Geometry check sheet. Reference: the model listing, model coordinates, mm. Round coordinates to 2 decimals unless told otherwise and drop trailing zeros. Order: outer loops, then holes, each group sorted by start corner. A loop starts at its lowest first (then second) coordinate and runs counter-clockwise, first axis right, second up. Notation, with made-up numbers: (33, 32) -> (61, 32) arc R20 ccw to (61, 66) -> close; hole circle Ø5 at (13.5, 12). An arc over 180 degrees is marked (long way). Use a Markdown table: item, result. Add a question column.
Item 1: Material ranges on probe 1 along X at (y, z) = (0.6, 0); probe 2 along Z at (x, y) = (-4.75, 0.5), recorded low to high. Write a range as [from, to].
Item 2: Mould release check, pull along Z, two halves, no side actions. Record for faces 1 (the cylindrical face through (-6.834, 0.887, -1.517)), 2 (the cylindrical face through (3.604, 0.99, 11.446)), 3 (the flat face through (-5.1, 0, 5.1)): pulls with the +Z half, pulls with the -Z half, needs draft (parallel to the pull), parting line crosses it, or undercut.
Item 3: Sectioned sample at B-B, the plane z = 0. Record the cut outline in (x, y).
Item 4: Gauge pin test, flat ends, axial feed: pin 1 Ø1 at (y, z) = (1.5, -7.5) entering from +X; pin 2 Ø8 at (x, z) = (2.5, -1) entering from +Y. Record the tip position at first contact, or that the pin passes through.
Item 5: Sectioned sample at A-A, the plane x = 0. Record the cut outline in (y, z).
from build123d import *

# Parameters (mm, degrees)
SKETCH1_R           = 12
BOSS_EXTRUDE1_DEPTH = 2
SKETCH2_R           = 7
CUT_EXTRUDE1_DEPTH  = 18.088007491
FILLET1_R           = 0.25


with BuildPart() as part:
    # Sketch1 → Boss-Extrude1 (new body)
    with BuildSketch(Plane(origin=(0, 0, 0), x_dir=(1, 0, 0), z_dir=(0, 1, 0))):
        with Locations(Location((0, 0, 0), (0, 0, 270))):
            Circle(SKETCH1_R)
    extrude(amount=BOSS_EXTRUDE1_DEPTH)

    # Sketch2 → Cut-Extrude1 (cut, through all)
    with BuildSketch(Plane(origin=(0, 2, 0), x_dir=(1, 0, 0), z_dir=(0, 1, 0))):
        with Locations(Location((0, 0, 0), (0, 0, 270))):
            Circle(SKETCH2_R)
    extrude(amount=-CUT_EXTRUDE1_DEPTH, mode=Mode.SUBTRACT)

    # Fillet1
    fillet1_edges = [part.edges().sort_by_distance(p)[0] for p in [
        (0, 0, -12),
        (0, 2, -12),
        (0, 2, -7),
    ]]
    fillet(fillet1_edges, radius=FILLET1_R)


solid = part.part
Found:
| question | item | result |
|---|---|---|
| 1 | probe 1 | x = [-12, -7], [7, 12] |
| 1 | probe 2 | z = [-11.02, -5.14], [5.14, 11.02] |
| 2 | face 1 | undercut |
| 2 | face 2 | parting line crosses it |
| 2 | face 3 | needs draft |
| 3 | outline | (-12, 0.25) arc R0.25 ccw to (-11.75, 0) -> (-7, 0) -> (-7, 1.75) arc R0.25 ccw to (-7.25, 2) -> (-11.75, 2) arc R0.25 ccw to (-12, 1.75) -> close; (7, 0) -> (11.75, 0) arc R0.25 ccw to (12, 0.25) -> (12, 1.75) arc R0.25 ccw to (11.75, 2) -> (7.25, 2) arc R0.25 ccw to (7, 1.75) -> close |
| 4 | pin 1 | stops at x = 9.75 |
| 4 | pin 2 | passes through |
| 5 | outline | (0, -11.75) arc R0.25 ccw to (0.25, -12) -> (1.75, -12) arc R0.25 ccw to (2, -11.75) -> (2, -7.25) arc R0.25 ccw to (1.75, -7) -> (0, -7) -> close; (0, 7) -> (1.75, 7) arc R0.25 ccw to (2, 7.25) -> (2, 11.75) arc R0.25 ccw to (1.75, 12) -> (0.25, 12) arc R0.25 ccw to (0, 11.75) -> close |
